Answer from the drawing. Dimensions are ordinates in mm from the lowest x, y and z of the part. A direction names the side the tool comes from. Give positions to 0.01 mm unless a question says otherwise; leave off trailing zeros. Loops run counter-clockwise (first coordinate to the right, second up) from the corner with the lowest first, then second, coordinate; pieces in that order, holes last.
Item 1: Each of these flat-tipped pins is pushed along its axis until it touches: pin 1 Ø1 at (y, z) = (28.5, 16) entering from -X; pin 2 Ø12 at (y, z) = (11, 30.5) entering from +X; pin 3 Ø12 at (x, y) = (12.5, 9) entering from -Z; pin 4 Ø12 at (x, z) = (26, 22.5) entering from -Y. Where does it stop, or does it pass through?
Item 2: Section C-C, the plane x = 13.5 is taken. Give the vertices of the cut face in (y, z), and give its area (3 significant figures).
Item 3: The mould has two halves that part along X. Classify the marked faces 1, 2 and 3: pulls with the +X half, pulls with the -X half, needs draft (parallel to the pull), parting line crosses it, or undercut.
Item 4: Section D-D, the plane z = 11 is taken. Give the vertices of the cut face in (x, y).
Item 5: A tool of negligible diameter and unlimited length cuts with its end or side. For the marked faces 4 and 5, from which of +Z, -Z, +X, -X, +Y, -Y can it reach the whole face along a straight path? Write none if from no direction.
Item 6: Consider line 1 along Y through (x, z) = (25, 47.5); line 2 along Y through (x, z) = (25, 31); line 3 along Z through (x, y) = (23.5, 4). Determine where each line is inside the solid, lowest interval first.
Item 7: Section A-A, the plane z = 33.5 is taken. Give the vertices of the cut face in (x, y).
Item 8: Section B-B, the plane y = 7 is taken. Give the vertices of the cut face in (x, z), and give its area (3 significant figures).
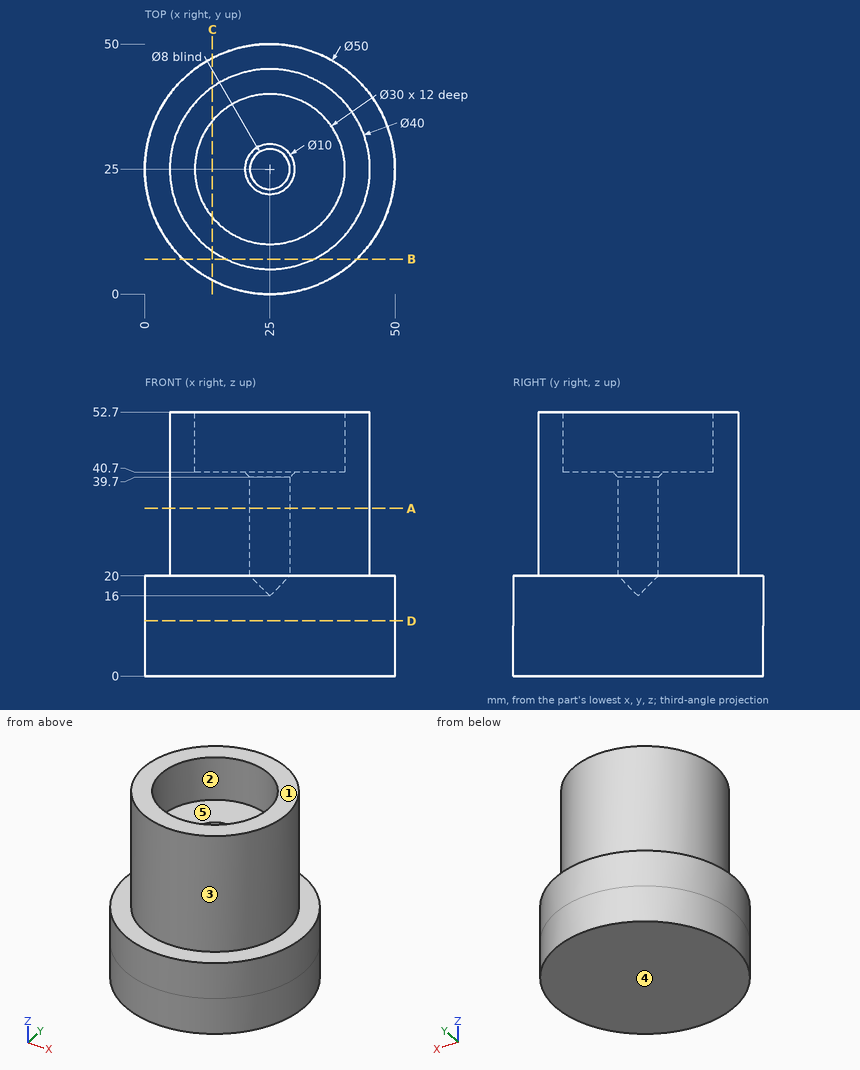
Worked answers:
1. pin 1: stops at x = 0.18
1. pin 2: stops at x = 43.33
1. pin 3: stops at z = 0
1. pin 4: stops at y = 0
2. outline: (2.8, 0) - (47.2, 0) - (47.2, 20) - (41.36, 20) - (41.36, 52.7) - (34.63, 52.7) - (34.63, 40.7) - (15.37, 40.7) - (15.37, 52.7) - (8.64, 52.7) - (8.64, 20) - (2.8, 20) - close
2. area: 1,730 mm2
3. face 1: needs draft
3. face 2: undercut
3. face 3: parting line crosses it
4. outline: circle Ø50 at (25, 25)
5. face 4: -Z, +X, -X, +Y, -Y
5. face 5: +Z
6. line 1: y = 5 to 10, 40 to 45
6. line 2: y = 5 to 21, 29 to 45
6. line 3: z = 0 to 20
7. outline: circle Ø40 at (25, 25); hole circle Ø8 at (25, 25)
8. outline: (7.65, 0) - (42.35, 0) - (42.35, 20) - (33.72, 20) - (33.72, 52.7) - (16.28, 52.7) - (16.28, 20) - (7.65, 20) - close
8. area: 1,260 mm2
